Read the model definition and answer for the solid it produces. Units are mm, in the model's axes. Face numbers are marked on the shaded views. Coordinates: 2 decimals unless noted, no trailing zeros. Order: outer loops, then holes, each group sorted by start corner. A loop starts at its lowest first (then second) coordinate and runs counter-clockwise, first axis right, second up. Notation, with made-up numbers: (54.5, 76) - (81.5, 76) arc R11 ccw to (81.5, 97) - close; hole circle Ø11 at (24, -23). An arc over 180 degrees is marked (long way). Write item = value, one per line.
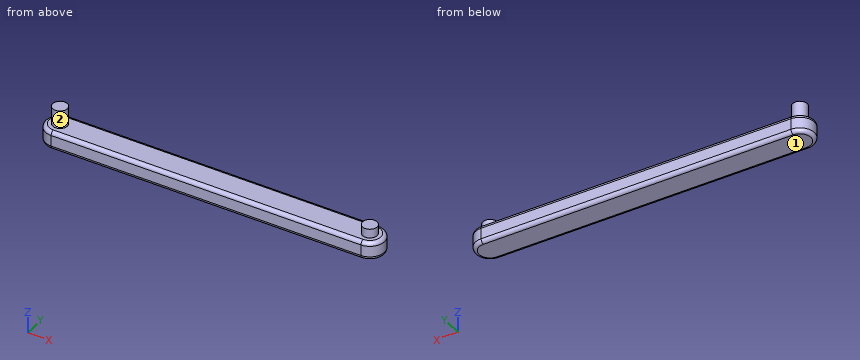
Autodesk Inventor part; units mm, degrees
ref_plane "Work Plane2" through (-8, 0, 0) normal (1, 0, 0) x (0, 1, 0)
ref_plane "XZ Plane" through (0, 0, 0) normal (0, 1, 0) x (-1, 0, 0)
ref_plane "XY Plane" through (0, 0, 0) normal (0, 0, 1) x (1, 0, 0)
sketch "Sketch1" plane through (0, 0, 0) normal (0, 0, 1) x (1, 0, 0)
  circle A0 centre (0, 0) radius 8
  dimension "d0" = 16
extrude "Extrusion1" add sketch "Sketch1" along normal blind 10
ref_plane "Work Plane1" through (8, 0, 0) normal (1, 0, 0) x (0, 1, 0)
sketch "Sketch2" plane through (8, 0, 0) normal (1, 0, 0) x (0, 1, 0)
  line L0 (-8, 0) -> (-8, 10)
  line L1 (8, 10) -> (-8, 10)
  line L2 (-8, 10) -> (-8, 0)
  line L3 (-8, 0) -> (8, 0)
  line L4 (8, 0) -> (8, 10)
  line L5 (8, 10) -> (-8, 0) construction
  line L6 (-8, 10) -> (8, 0) construction
  point P0 (0, 0)
  point P1 (0, 5)
extrude "Extrusion2" add sketch "Sketch2" along normal blind 162 and the other way blind 8
sketch "Sketch3" plane through (0, 0, 10) normal (0, 0, 1) x (1, 0, 0)
  arc A0 (0, 8) -> (0, -8) centre (0, 0) ccw
  line L0 (0, 0) -> (170, 0)
  line L1 (170, -8) -> (0, -8)
  line L2 (0, 0) -> (170, 0) construction
  line L3 (170, 8) -> (170, -8)
  circle A1 centre (170, 0) radius 8
  dimension "d8" = 170
  dimension "d9" = 0
extrude "Extrusion3" add sketch "Sketch3" against normal blind 10
ref_plane "Work Plane2" through (-8, 0, 0) normal (1, 0, 0) x (0, 1, 0)
sketch "Sketch4" plane through (-8, 0, 0) normal (1, 0, 0) x (0, 1, 0)
  line L0 (-8, 0) -> (-8, 10)
  line L1 (8, 7.5) -> (-8, 7.5)
  line L2 (-8, 7.5) -> (-8, 2.5)
  line L3 (-8, 2.5) -> (8, 2.5)
  line L4 (8, 2.5) -> (8, 7.5)
  line L5 (8, 7.5) -> (-8, 2.5) construction
  line L6 (-8, 7.5) -> (8, 2.5) construction
  line L7 (8, 10) -> (-8, 10)
  line L8 (8, 0) -> (8, 10)
  line L9 (-8, 10) -> (-8, 0)
  line L10 (-8, 0) -> (8, 0)
  point P0 (0, 0)
  point P1 (0, 5)
  dimension "d13" = 5
extrude "Extrusion4" [suppressed]
sketch "Sketch5" plane through (0, -8, 7.5) normal (0, 0, 1) x (1, 0, 0)
  circle A0 centre (0, 8) radius 4
  dimension "d16" = 8
extrude "Extrusion5" [suppressed]
sketch "Sketch6" plane through (0, 0, 10) normal (0, 0, 1) x (1, 0, 0)
  arc A0 (170, -8) -> (170, 8) centre (170, 0) ccw
  circle A1 centre (170, 0) radius 4
  point P0 (0, 0)
  dimension "d21" = 8
extrude "Extrusion6" add sketch "Sketch6" along normal blind 5
sketch "Sketch7" plane through (0, 0, 10) normal (0, 0, 1) x (1, 0, 0)
  circle A0 centre (0, 0) radius 4
  dimension "d24" = 8
extrude "Extrusion7" add sketch "Sketch7" along normal blind 10
fillet "Fillet1" radius 2 8 edges at (178, 0, 0) (85, -8, 0) (-8, 0, 0) (85, 8, 0) (178, 0, 10) (85, -8, 10) (-8, 0, 10) (85, 8, 10)
properties part number "Acoplador" material "Iron, Ductile"
1) Straight lines are drawn through the part: line 1 along X through (y, z) = (0.25, 15.5); line 2 along Z through (x, y) = (151, -5); line 3 along X through (y, z) = (3, 14). For each, find the intervals that lie inside material, in ascending order. Write a range as from..to.
Returned:
line_1 = -3.99..3.99
line_2 = 0..10
line_3 = -2.65..2.65, 167.35..172.65
2) The part is cut by section B-B (x = 102). Determine the outline of the cut face in (y, z).
Returned:
outline = (-8, 2) arc R2 ccw to (-6, 0) - (6, 0) arc R2 ccw to (8, 2) - (8, 8) arc R2 ccw to (6, 10) - (-6, 10) arc R2 ccw to (-8, 8) - close
3) Determine the mould class of the marked faces 1 and 2 for opening direction X: pulls with the +X half, pulls with the -X half, needs draft (parallel to the pull), parting line crosses it, or undercut.
Returned:
face_1 = needs draft
face_2 = undercut
4) Flat-ended cylindrical pins translate along their axes: pin 1 Ø4 at (x, y) = (169.5, -1.5) entering from +Z; pin 2 Ø3 at (x, z) = (36, 10) entering from -Y; pin 3 Ø1.5 at (y, z) = (5.5, 3) entering from +X. Find the tip coordinate at first contact, or state that the pin passes through.
Returned:
pin_1 = 15
pin_2 = -7.94
pin_3 = 176.44
5) The part is cut by section A-A (y = 0). Determine the outline of the cut face in (x, z).
Returned:
outline = (-8, 2) arc R2 ccw to (-6, 0) - (176, 0) arc R2 ccw to (178, 2) - (178, 8) arc R2 ccw to (176, 10) - (174, 10) - (174, 15) - (166, 15) - (166, 10) - (4, 10) - (4, 20) - (-4, 20) - (-4, 10) - (-6, 10) arc R2 ccw to (-8, 8) - close
6) The part is cut by section C-C (z = 18). Determine the outline of the cut face in (x, y), and give its area (3 significant figures).
Returned:
outline = circle Ø8 at (0, 0)
area = 50.3 mm^2
